Model file for the job. Use its own axes, mm. A direction names the side the tool comes from. Give positions to 0.01 mm unless a question says otherwise; leave off trailing zeros. Loops run counter-clockwise (first coordinate to the right, second up) from the corner with the lowest first, then second, coordinate; pieces in that order, holes last. Notation, with made-up numbers: (73.25, 30.25) - (111.25, 30.25) arc R37 ccw to (111.25, 69.25) - close; hole circle Ø11 at (15, 79.5). An arc over 180 degrees is marked (long way). Answer as CSV lines item,"result". Start each with the question number.
Item 1: Drill centre lines: L1, parallel to Y at x = 238, z = 29; L2, parallel to X at y = 1, z = 57.5; L3, parallel to X at y = 2.5, z = 43. Where is each one in solid material? Low to high. Write a range as from..to.
Item 2: Pull direction X, two halves, no side cores. Call faces 1 (the flat face through (242, 5, 0)), 2 (the cylindrical face through (235.95, 2.81, 30.52)), 3 (the conical face through (240.548, 2.743, 55.779)): pulls with the +X half, pulls with the -X half, needs draft (parallel to the pull), parting line crosses it, or undercut.
Item 3: Saw through at B-B on z = 24. Give the cut face in (x, y) (1 decimal), plus the area to 3 significant figures.
Item 4: Pin check, flat tips, straight feed: pin 1 (4 mm diameter, centred on y = 5, z = 17, fed in from -X); pin 2 (4 mm diameter, centred on x = 243.5, z = 15.5, fed in from +Y); pin 3 (2 mm diameter, centred on x = 240.71, y = 2.6, fed in from +Z). Stop position of each tip, or through.
Item 5: Tool access for faces 4 (the cylindrical face through (239.554, 2.117, 58.865)), 5 (the cylindrical face through (238.61, 2.69, 7.1)), 6 (the cylindrical face through (240.04, 1.54, 28.49)): list every direction of +Z, -Z, +X, -X, +Y, -Y with a clear straight run to the whole face (end or side of a thin tool).
Item 6: Saw through at A-A on z = 8. Give the cut face in (x, y) (1 decimal).
from build123d import *

# Parameters (mm, degrees)
ESBO_O1_R                                      = 4.7625
RESSALTO_EXTRUS_O1_DEPTH                       = 61.4
FURO_ROSCADO_DE_M5X0_81_D                      = 4.2
FURO_ROSCADO_DE_M5X0_81_DEPTH                  = 14
FURO_ROSCADO_DE_M5X0_81_TIP                    = 1.2618073
FILETE1_R                                      = 0.5
BROCA_DE_ROSQUEAR_PARA_TARRAXA_DE_M3X0_5_D     = 2.5
BROCA_DE_ROSQUEAR_PARA_TARRAXA_DE_M3X0_5_DEPTH = 5
BROCA_DE_ROSQUEAR_PARA_TARRAXA_DE_M3X0_5_TIP   = 0.751075774
BROCA_DE_ROSQUEAR_PARA_TARRAXA_DE_M3_2_D       = 2.5
BROCA_DE_ROSQUEAR_PARA_TARRAXA_DE_M3_2_DEPTH   = 10
BROCA_DE_ROSQUEAR_PARA_TARRAXA_DE_M3_2_TIP     = 0.751075774


with BuildPart() as part:
    # Esboço1 → Ressalto-extrusão1 (new body)
    with BuildSketch(Plane.XY):
        with Locations((240.708388302, 2.596082859)):
            Circle(ESBO_O1_R)
    extrude(amount=RESSALTO_EXTRUS_O1_DEPTH)

    # Furo roscado de M5x0.81
    with Locations(Plane(origin=(0, 0, 0), x_dir=(-1, 0, 0), z_dir=(0, 0, -1))):
        with Locations((-240.708388302, 2.596082859)):
            Hole(FURO_ROSCADO_DE_M5X0_81_D / 2, depth=FURO_ROSCADO_DE_M5X0_81_DEPTH)
            with Locations((0, 0, -(FURO_ROSCADO_DE_M5X0_81_DEPTH + FURO_ROSCADO_DE_M5X0_81_TIP / 2))):  # 118° drill point
                Cone(0, FURO_ROSCADO_DE_M5X0_81_D / 2, FURO_ROSCADO_DE_M5X0_81_TIP, mode=Mode.SUBTRACT)

    # Filete1
    filete1_edges = [part.edges().sort_by_distance(p)[0] for p in [
        (235.945888302, 2.596082859, 0),
    ]]
    fillet(filete1_edges, radius=FILETE1_R)

    # Broca de rosquear para tarraxa de M3x0.5
    with Locations(Plane.XY.offset(61.4)):
        with Locations((240.708388302, 2.596082859)):
            Hole(BROCA_DE_ROSQUEAR_PARA_TARRAXA_DE_M3X0_5_D / 2, depth=BROCA_DE_ROSQUEAR_PARA_TARRAXA_DE_M3X0_5_DEPTH)
            with Locations((0, 0, -(BROCA_DE_ROSQUEAR_PARA_TARRAXA_DE_M3X0_5_DEPTH + BROCA_DE_ROSQUEAR_PARA_TARRAXA_DE_M3X0_5_TIP / 2))):  # 118° drill point
                Cone(0, BROCA_DE_ROSQUEAR_PARA_TARRAXA_DE_M3X0_5_D / 2, BROCA_DE_ROSQUEAR_PARA_TARRAXA_DE_M3X0_5_TIP, mode=Mode.SUBTRACT)

    # Broca de rosquear para tarraxa de M3 2
    with Locations(Plane(origin=(236.819403783, 5.345120084, 28.431873204), x_dir=(-0.577225664074, -0.81658467579, 0), z_dir=(-0.81658467579, 0.577225664074, 0))):
        with Locations((0, 0)):
            Hole(BROCA_DE_ROSQUEAR_PARA_TARRAXA_DE_M3_2_D / 2, depth=BROCA_DE_ROSQUEAR_PARA_TARRAXA_DE_M3_2_DEPTH)
            with Locations((0, 0, -(BROCA_DE_ROSQUEAR_PARA_TARRAXA_DE_M3_2_DEPTH + BROCA_DE_ROSQUEAR_PARA_TARRAXA_DE_M3_2_TIP / 2))):  # 118° drill point
                Cone(0, BROCA_DE_ROSQUEAR_PARA_TARRAXA_DE_M3_2_D / 2, BROCA_DE_ROSQUEAR_PARA_TARRAXA_DE_M3_2_TIP, mode=Mode.SUBTRACT)


solid = part.part
Responses:
1,L1,"-1.32..3.15, 5.87..6.51"
1,L2,"236.22..245.2"
1,L3,"235.95..245.47"
2,face 1,"needs draft"
2,face 2,"parting line crosses it"
2,face 3,"undercut"
3,outline,"circle Ø9.5 at (240.7, 2.6)"
3,area,"71.3 mm2"
4,pin 1,"x = 235.96"
4,pin 2,"y = 7.29"
4,pin 3,"z = 56.25"
5,face 4,"+Z"
5,face 5,"-Z"
5,face 6,"none"
6,outline,"circle Ø9.5 at (240.7, 2.6); hole circle Ø4.2 at (240.7, 2.6)"
